Read the model definition and answer for the solid it produces. Units are mm, in the model's axes. Round coordinates to 2 decimals unless told otherwise and drop trailing zeros. Write each loop counter-clockwise with the first axis right and the second up, starting at its lowest first coordinate (ties: lowest second). Pieces come first, ordered by that corner, then holes.
from build123d import *

# Parameters (mm, degrees)
CROQUIS1_W                   = 2.54
CROQUIS1_H                   = 2.54
CROQUIS1_W_2                 = 0.6
CROQUIS1_H_2                 = 0.6
SALIENTE_EXTRUIR1_DEPTH      = 2.54
SALIENTE_EXTRUIR2_DEPTH      = 6
SALIENTE_EXTRUIR2_DEPTH_BACK = 5.5
CROQUIS2_W                   = 0.6
CROQUIS2_H                   = 0.6


with BuildPart() as part:
    # Croquis1 → Saliente-Extruir1 (new body)
    with BuildSketch(Plane.XY):
        Rectangle(CROQUIS1_W, CROQUIS1_H)
        Rectangle(CROQUIS1_W_2, CROQUIS1_H_2, mode=Mode.SUBTRACT)
    extrude(amount=SALIENTE_EXTRUIR1_DEPTH)

    # Croquis2 → Saliente-Extruir2 (add, two sides: drawn at the far end of the back side and taken through both)
    with BuildSketch(Plane.XY.offset(2.54).offset(-SALIENTE_EXTRUIR2_DEPTH_BACK)):
        Rectangle(CROQUIS2_W, CROQUIS2_H)
    extrude(amount=SALIENTE_EXTRUIR2_DEPTH + SALIENTE_EXTRUIR2_DEPTH_BACK)


solid = part.part
Q1. Flat-ended cylindrical pins translate along their axes: pin 1 Ø1.5 at (x, z) = (0.5, 6.5) entering from +Y; pin 2 Ø0.7 at (x, z) = (0, 5) entering from -Y; pin 3 Ø0.5 at (y, z) = (0, 5.5) entering from +X. Find the tip coordinate at first contact, or state that the pin passes through.
Verdict:
pin 1: stops at y = 0.3
pin 2: stops at y = -0.3
pin 3: stops at x = 0.3
Q2. Section C-C (x = 1.05) is taken. Determine the outline of the cut face in (y, z).
Verdict:
outline: (-1.27, 0) - (1.27, 0) - (1.27, 2.54) - (-1.27, 2.54) - close
Q3. Straight lines are drawn through the part: probe 1 along Z at (x, y) = (-0.5, -0.7); probe 2 along X at (y, z) = (0.25, -1). For each, find the intervals that lie inside material, in ascending order.
Verdict:
probe 1: z = 0 to 2.54
probe 2: x = -0.3 to 0.3
Q4. Section A-A (y = -0.1) is taken. Determine the outline of the cut face in (x, z).
Verdict:
outline: (-1.27, 0) - (-0.3, 0) - (-0.3, -2.96) - (0.3, -2.96) - (0.3, 0) - (1.27, 0) - (1.27, 2.54) - (0.3, 2.54) - (0.3, 8.54) - (-0.3, 8.54) - (-0.3, 2.54) - (-1.27, 2.54) - close
Q5. Section B-B (z = 6.75) is taken. Determine the outline of the cut face in (x, y).
Verdict:
outline: (-0.3, -0.3) - (0.3, -0.3) - (0.3, 0.3) - (-0.3, 0.3) - close
